```python
from build123d import *

# Parameters (mm, degrees)
SKETCH_1_W               = 120
SKETCH_1_H               = 100
EXTRUDE_1_DEPTH          = 3
FILLET_1_R               = 5
SKETCH_4_R               = 2.1
CUT_EXTRUDE_2_DEPTH      = 79.160092119
PATTERN_LINEAR_1_COUNT   = 3
PATTERN_LINEAR_1_PITCH   = 40
MIRROR_1_COPY_1_SKETCH_R = 2.1
MIRROR_1_COPY_1_DEPTH    = 79.160092119
MIRROR_1_COPY_2_SKETCH_R = 2.1
MIRROR_1_COPY_2_DEPTH    = 79.160092119


with BuildPart() as part:
    # 草图1 → 凸台-拉伸1 (new body)
    with BuildSketch(Plane(origin=(0, 0, 0), x_dir=(1, 0, 0), z_dir=(0, 1, 0))):
        Rectangle(SKETCH_1_W, SKETCH_1_H)
    extrude(amount=EXTRUDE_1_DEPTH)

    # 圆角1
    fillet_1_edges = [part.edges().sort_by_distance(p)[0] for p in [
        (60, 1.5, 50),
        (-60, 1.5, 50),
        (-60, 1.5, -50),
        (60, 1.5, -50),
    ]]
    fillet(fillet_1_edges, radius=FILLET_1_R)

    # 草图4 → 切除-拉伸2 (cut, through all)
    with BuildSketch(Plane(origin=(0, 3, 0), x_dir=(1, 0, 0), z_dir=(0, 1, 0))):
        with Locations(Location((50, 40, 0), (0, 0, 270))):
            Circle(SKETCH_4_R)
    cut_extrude_2 = extrude(amount=-CUT_EXTRUDE_2_DEPTH, mode=Mode.SUBTRACT)

    # 阵列(线性)1: 切除-拉伸2 ×3
    with Locations(*[(0, 0, i * PATTERN_LINEAR_1_PITCH) for i in range(1, PATTERN_LINEAR_1_COUNT)]):
        add(cut_extrude_2, mode=Mode.SUBTRACT)

    # 镜向1: 切除-拉伸2 across plane
    add(cut_extrude_2.mirror(Plane(origin=(0, 0, 0), x_dir=(0, 0, 1), z_dir=(1, 0, 0))), mode=Mode.SUBTRACT)

    # 镜向1 copy 1 sketch → 镜向1 copy 1 (cut, through all)
    with BuildSketch(Plane(origin=(0, 3, 40), x_dir=(-1, 0, 0), z_dir=(0, 1, 0))):
        with Locations((50, -40)):
            Circle(MIRROR_1_COPY_1_SKETCH_R)
    extrude(amount=-MIRROR_1_COPY_1_DEPTH, mode=Mode.SUBTRACT)

    # 镜向1 copy 2 sketch → 镜向1 copy 2 (cut, through all)
    with BuildSketch(Plane(origin=(0, 3, 80), x_dir=(-1, 0, 0), z_dir=(0, 1, 0))):
        with Locations((50, -40)):
            Circle(MIRROR_1_COPY_2_SKETCH_R)
    extrude(amount=-MIRROR_1_COPY_2_DEPTH, mode=Mode.SUBTRACT)


solid = part.part
```
Could you check a few things on this model? Use its own coordinates, in mm. Give positions to 0.01 mm unless a question says otherwise; leave off trailing zeros. Loops run counter-clockwise (first coordinate to the right, second up) from the corner with the lowest first, then second, coordinate; pieces in that order, holes last. Notation, with made-up numbers: (-26.5, -31.75) - (-12.5, -31.75) arc R25 cw to (-12.5, -3.75) - close; hole circle Ø8 at (-11, 45.5). An arc over 180 degrees is marked (long way). Use one line per item in the form item = value.
1. Thinking about a two-plate mould opening in X: for faces 1 (the face through (59, 2, -48)), 2 (the face through (-59, 2, 48)), 3 (the face through (-51.94, 1.52, -0.8)), 4 (the face through (-1, 3, -1)), which applies, released by +X, released by -X, zero draft, split by the parting line, or undercut?
Response values:
face_1 = released by +X
face_2 = released by -X
face_3 = undercut
face_4 = zero draft
2. I want a section at A-A (z = -40). Please give me the cut outline in (x, y), and give its area (3 significant figures).
Response values:
outline = (-60, 0) - (-52.1, 0) - (-52.1, 3) - (-60, 3) - close; (-47.9, 0) - (47.9, 0) - (47.9, 3) - (-47.9, 3) - close; (52.1, 0) - (60, 0) - (60, 3) - (52.1, 3) - close
area = 335 mm²
3. I want a section at B-B (x = -50). Please give me the cut outline in (y, z).
Response values:
outline = (0, -50) - (3, -50) - (3, -42.1) - (0, -42.1) - close; (0, -37.9) - (3, -37.9) - (3, -2.1) - (0, -2.1) - close; (0, 2.1) - (3, 2.1) - (3, 37.9) - (0, 37.9) - close; (0, 42.1) - (3, 42.1) - (3, 50) - (0, 50) - close
4. I'm going to push a flat-ended pin straight in: pin 1 Ø2.5 at (x, z) = (50, 40) entering from -Y. Where does the tip first touch, or does it pass through?
Response values:
pin_1 = through
